from build123d import *

# Parameters (mm, degrees)
SKETCH1_R           = 44.45
SKETCH1_R_2         = 40.64
BOSS_EXTRUDE1_DEPTH = 393.7
SKETCH3_R           = 40.64
BOSS_EXTRUDE2_DEPTH = 25.4
SKETCH4_R           = 34.925
BOSS_EXTRUDE3_DEPTH = 25.4
SKETCH6_R           = 40.64
BOSS_EXTRUDE4_DEPTH = 25.4
SKETCH7_R           = 34.925
BOSS_EXTRUDE5_DEPTH = 25.4
SKETCH9_R           = 17.78
CUT_EXTRUDE1_DEPTH  = 152.4


with BuildPart() as part:
    # Sketch1 → Boss-Extrude1 (new body)
    with BuildSketch(Plane(origin=(0, 0, 0), x_dir=(1, 0, 0), z_dir=(0, 1, 0))):
        Circle(SKETCH1_R)
        Circle(SKETCH1_R_2, mode=Mode.SUBTRACT)
    extrude(amount=BOSS_EXTRUDE1_DEPTH)

    # Sketch3 → Boss-Extrude2 (add)
    with BuildSketch(Plane(origin=(0, 355.6, 0), x_dir=(1, 0, 0), z_dir=(0, 1, 0))):
        Circle(SKETCH3_R)
    extrude(amount=BOSS_EXTRUDE2_DEPTH)

    # Sketch4 → Boss-Extrude3 (add)
    with BuildSketch(Plane(origin=(0, 381, 0), x_dir=(1, 0, 0), z_dir=(0, 1, 0))):
        Circle(SKETCH4_R)
    extrude(amount=BOSS_EXTRUDE3_DEPTH)

    # Sketch6 → Boss-Extrude4 (add)
    with BuildSketch(Plane(origin=(0, 38.1, 0), x_dir=(-1, 0, 0), z_dir=(0, -1, 0))):
        Circle(SKETCH6_R)
    extrude(amount=BOSS_EXTRUDE4_DEPTH)

    # Sketch7 → Boss-Extrude5 (add)
    with BuildSketch(Plane.XZ.offset(-12.7)):
        Circle(SKETCH7_R)
    extrude(amount=BOSS_EXTRUDE5_DEPTH)

    # Sketch9 → Cut-Extrude1 (cut)
    with BuildSketch(Plane(origin=(0, 406.4, 0), x_dir=(1, 0, 0), z_dir=(0, 1, 0))):
        Circle(SKETCH9_R)
    extrude(amount=-CUT_EXTRUDE1_DEPTH, mode=Mode.SUBTRACT)


solid = part.part
Check sheet for the modelled part. Datum: model origin and axes. Units: mm. A direction names the side the tool comes from. Coordinates: 2 decimals unless noted, no trailing zeros. Write each loop counter-clockwise with the first axis right and the second up, starting at its lowest first coordinate (ties: lowest second). Pieces come first, ordered by that corner, then holes.
Item 1: Mould release check, pull along Y, two halves, no side actions. Record for faces 1 (the face through (-3.85, 381.36, 17.36)), 2 (the face through (17.9, 381, -30.3)), 3 (the face through (-5.291, 194.628, -40.294)): released by +Y, released by -Y, zero draft, split by the parting line, or undercut.
Numbers:
face 1: zero draft
face 2: released by +Y
face 3: undercut
Item 2: Cross-section at C-C on z = 23.5. Record the boundary of the cut face in (x, y).
Numbers:
outline: (-37.73, 0) - (-33.16, 0) - (-33.16, 12.7) - (-25.84, 12.7) - (-25.84, -12.7) - (25.84, -12.7) - (25.84, 12.7) - (33.16, 12.7) - (33.16, 0) - (37.73, 0) - (37.73, 393.7) - (33.16, 393.7) - (33.16, 381) - (25.84, 381) - (25.84, 406.4) - (-25.84, 406.4) - (-25.84, 381) - (-33.16, 381) - (-33.16, 393.7) - (-37.73, 393.7) - close; hole (-33.16, 38.1) - (33.16, 38.1) - (33.16, 355.6) - (-33.16, 355.6) - close
Item 3: Depth check by flat-ended pin: pin 1 Ø4 at (x, y) = (-16, 253) entering from +Z; pin 2 Ø12 at (x, y) = (34.5, 139.5) entering from -Z; pin 3 Ø6 at (x, y) = (-13.5, 216) entering from +Z. Enter the tip coordinate at first touch or a pass-through.
Numbers:
pin 1: stops at z = 42.19
pin 2: stops at z = -34.11
pin 3: stops at z = 43.19
Item 4: Access from +Z, -Z, +X, -X, +Y, -Y to the whole of each face (thin tool, end or side, straight path). Record for faces 4 (the face through (20, 393.7, 36)), 5 (the face through (0, -12.7, 0)), 6 (the face through (-27.715, 0.178, -21.251)), 7 (the face through (1, 38.1, -1)).
Numbers:
face 4: +Y
face 5: +Z, -Z, +X, -X, -Y
face 6: -Y
face 7: none
Item 5: Cross-section at A-A on z = 0. Record the boundary of the cut face in (x, y) (3 decimals).
Numbers:
outline: (-44.45, 0) - (-40.64, 0) - (-40.64, 12.7) - (-34.925, 12.7) - (-34.925, -12.7) - (34.925, -12.7) - (34.925, 12.7) - (40.64, 12.7) - (40.64, 0) - (44.45, 0) - (44.45, 393.7) - (40.64, 393.7) - (40.64, 381) - (34.925, 381) - (34.925, 406.4) - (17.78, 406.4) - (17.78, 355.6) - (40.64, 355.6) - (40.64, 38.1) - (-40.64, 38.1) - (-40.64, 355.6) - (-17.78, 355.6) - (-17.78, 406.4) - (-34.925, 406.4) - (-34.925, 381) - (-40.64, 381) - (-40.64, 393.7) - (-44.45, 393.7) - close
Item 6: Cross-section at D-D on y = 91.5. Record the boundary of the cut face in (x, z), then the cut area to 3 significant figures.
Numbers:
outline: circle Ø88.9 at (0, 0); hole circle Ø81.28 at (0, 0)
area: 1,020 mm2
Item 7: Cross-section at B-B on x = 0. Record the boundary of the cut face in (y, z) (3 decimals).
Numbers:
outline: (-12.7, -34.925) - (12.7, -34.925) - (12.7, -40.64) - (0, -40.64) - (0, -44.45) - (393.7, -44.45) - (393.7, -40.64) - (381, -40.64) - (381, -34.925) - (406.4, -34.925) - (406.4, -17.78) - (355.6, -17.78) - (355.6, -40.64) - (38.1, -40.64) - (38.1, 40.64) - (355.6, 40.64) - (355.6, 17.78) - (406.4, 17.78) - (406.4, 34.925) - (381, 34.925) - (381, 40.64) - (393.7, 40.64) - (393.7, 44.45) - (0, 44.45) - (0, 40.64) - (12.7, 40.64) - (12.7, 34.925) - (-12.7, 34.925) - close
Item 8: Scan lines: probe 1 along X at (y, z) = (384, 0) (3 decimals); probe 2 along Y at (x, z) = (10.5, -29). Record each from-to range of solid material in increasing order.
Numbers:
probe 1: x = -44.45 to -40.64, -34.925 to -17.78, 17.78 to 34.925, 40.64 to 44.45
probe 2: y = -12.7 to 38.1, 355.6 to 406.4
